Read the model definition and answer for the solid it produces. Units are mm, in the model's axes. A direction names the side the tool comes from. Coordinates: 2 decimals unless noted, no trailing zeros. Write each loop counter-clockwise with the first axis right and the second up, starting at its lowest first coordinate (ties: lowest second). Pieces come first, ordered by that corner, then holes.
(1) Find the intervals of material crossed by probe 1 along Z at (x, y) = (0, 2.1); probe 2 along Y at (x, z) = (-3.75, -6.5), in increasing order.
(2) Given pin 1 (2.5 mm diameter, centred on x = -0.5, z = 1, fed in from -Y); pin 2 (5 mm diameter, centred on y = -9.5, z = -0.5, fed in from +X); pin 3 (1.5 mm diameter, centred on y = -12, z = -0.5, fed in from -X); pin 4 (1.3 mm diameter, centred on x = 0, z = 0, fed in from -Y), each flat-ended and moving along its own axis, determine where each tip first touches the part or whether it passes through.
(3) Which of the six approach directions +Z, -Z, +X, -X, +Y, -Y give full straight-line access (tool end or side, diameter ignored) to faces 1 (the cylindrical face through (-5.467, -6.409, 3.17)), 2 (the flat face through (-2.95, -6.41, -5.05)), 3 (the flat face through (1, 0, -1)), 4 (the flat face through (5.85, -6, 0))?
(4) Section C-C on x = 3.25 is taken. Write down the section's boundary in (y, z), then the cut area to 3 significant figures.
(5) The mould has two halves that part along X. Classify faces 5 (the cylindrical face through (-5.48, -6.41, -3.15)), 6 (the flat face through (2.9, -6.41, -5.08)), 7 (the cylindrical face through (1, 1.52, -0.32)): +X half, -X half, draft (parallel to the pull), parting line (faces both ways), or undercut.
(6) Section A-A on z = 0 is taken. Write down the section's boundary in (x, y), then the cut area to 3 significant figures.
(7) Section B-B on y = -3.25 is taken. Write down the section's boundary in (x, z).
(8) Section D-D on y = -14 is taken. Write down the section's boundary in (x, z), then the cut area to 3 significant figures.
from build123d import *

# Parameters (mm, degrees)
SKETCH1_R           = 8
BOSS_EXTRUDE1_DEPTH = 3
BOSS_EXTRUDE2_DEPTH = 15
CHAMFER1_SIZE       = 2
SKETCH10_R          = 2.5
CUT_EXTRUDE1_DEPTH  = 15
SKETCH11_R          = 1.05
CUT_EXTRUDE3_DEPTH  = 19


with BuildPart() as part:
    # Sketch1 → Boss-Extrude1 (new body)
    with BuildSketch(Plane(origin=(0, 0, 0), x_dir=(1, 0, 0), z_dir=(0, 1, 0))):
        Circle(SKETCH1_R)
    extrude(amount=BOSS_EXTRUDE1_DEPTH)

    # Sketch9 → Boss-Extrude2 (add)
    with BuildSketch(Plane.XZ):
        with BuildLine():
            ThreePointArc((-0.853786588, -6.262064233), (0, -6.32), (0.853786588, -6.262064233))
            Line((0.853786588, -6.262064233), (4.996213412, -3.870432991))
            ThreePointArc((4.996213412, -3.870432991), (5.473280552, -3.16), (5.85, -2.391631242))
            Line((5.85, -2.391631242), (5.85, 2.391631242))
            ThreePointArc((5.85, 2.391631242), (5.473280552, 3.16), (4.996213412, 3.870432991))
            Line((4.996213412, 3.870432991), (0.853786588, 6.262064233))
            ThreePointArc((0.853786588, 6.262064233), (0, 6.32), (-0.853786588, 6.262064233))
            Line((-0.853786588, 6.262064233), (-4.996213412, 3.870432991))
            ThreePointArc((-4.996213412, 3.870432991), (-5.473280552, 3.16), (-5.85, 2.391631242))
            Line((-5.85, 2.391631242), (-5.85, -2.391631242))
            ThreePointArc((-5.85, -2.391631242), (-5.473280552, -3.16), (-4.996213412, -3.870432991))
            Line((-4.996213412, -3.870432991), (-0.853786588, -6.262064233))
        make_face()
    extrude(amount=BOSS_EXTRUDE2_DEPTH)

    # Chamfer1
    chamfer1_edges = [part.edges().sort_by_distance(p)[0] for p in [
        (2.925, -15, -5.066248612),
        (5.473280552, -15, -3.16),
        (5.85, -15, 0),
        (5.473280552, -15, 3.16),
        (2.925, -15, 5.066248612),
        (0, -15, 6.32),
        (-2.925, -15, 5.066248612),
        (-5.473280552, -15, 3.16),
        (-5.85, -15, 0),
        (-5.473280552, -15, -3.16),
        (-2.925, -15, -5.066248612),
        (0, -15, -6.32),
    ]]
    chamfer(chamfer1_edges, length=CHAMFER1_SIZE)

    # Sketch10 → Cut-Extrude1 (cut)
    with BuildSketch(Plane.XZ.offset(15)):
        Circle(SKETCH10_R)
    extrude(amount=-CUT_EXTRUDE1_DEPTH, mode=Mode.SUBTRACT)

    # Sketch11 → Cut-Extrude3 (cut, through all)
    with BuildSketch(Plane(origin=(0, 3, 0), x_dir=(1, 0, 0), z_dir=(0, 1, 0))):
        Circle(SKETCH11_R)
    extrude(amount=-CUT_EXTRUDE3_DEPTH, mode=Mode.SUBTRACT)


solid = part.part
Response:
1. probe 1: z = -8 to -1.05, 1.05 to 8
1. probe 2: y = 0 to 3
2. pin 1: stops at y = 0
2. pin 2: stops at x = 5.85
2. pin 3: stops at x = -5.85
2. pin 4: passes through
3. face 1: +Z, -X, -Y
3. face 2: -Z, -X, -Y
3. face 3: -Y
3. face 4: +Z, -Z, +X, -Y
4. outline: (-15, -2.57) - (-13, -4.88) - (0, -4.88) - (0, -7.31) - (3, -7.31) - (3, 7.31) - (0, 7.31) - (0, 4.88) - (-13, 4.88) - (-15, 2.57) - close
4. area: 186 mm2
5. face 5: -X half
5. face 6: +X half
5. face 7: undercut
6. outline: (-8, 0) - (-5.85, 0) - (-5.85, -13) - (-3.85, -15) - (-2.5, -15) - (-2.5, 0) - (-1.05, 0) - (-1.05, 3) - (-8, 3) - close; (1.05, 0) - (2.5, 0) - (2.5, -15) - (3.85, -15) - (5.85, -13) - (5.85, 0) - (8, 0) - (8, 3) - (1.05, 3) - close
6. area: 138 mm2
7. outline: (-5.85, -2.39) arc R6.32 ccw to (-5, -3.87) - (-0.85, -6.26) arc R6.32 ccw to (0.85, -6.26) - (5, -3.87) arc R6.32 ccw to (5.85, -2.39) - (5.85, 2.39) arc R6.32 ccw to (5, 3.87) - (0.85, 6.26) arc R6.32 ccw to (-0.85, 6.26) - (-5, 3.87) arc R6.32 ccw to (-5.85, 2.39) - close; hole circle Ø5 at (0, 0)
8. outline: (-4.85, -2.19) arc R5.32 ccw to (-4.32, -3.11) - (-0.53, -5.29) arc R5.32 ccw to (0.53, -5.29) - (4.32, -3.11) arc R5.32 ccw to (4.85, -2.19) - (4.85, 2.19) arc R5.32 ccw to (4.32, 3.11) - (0.53, 5.29) arc R5.32 ccw to (-0.53, 5.29) - (-4.32, 3.11) arc R5.32 ccw to (-4.85, 2.19) - close; hole circle Ø5 at (0, 0)
8. area: 61.0 mm2
